Input: part model. Units: mm. Frame: model coordinates. A direction names the side the tool comes from. Coordinates: 2 decimals unless noted, no trailing zeros. Order: outer loops, then holes, each group sorted by start corner. A loop starts at its lowest first (then second) coordinate and runs counter-clockwise, first axis right, second up. Notation, with made-up numbers: (-19, 58) -> (0, 58) arc R20 cw to (0, 71) -> close; hole circle Ø6 at (55, 0.25). An arc over 180 degrees is marked (long way). Write each question's results on one line, items separated by ' | '.
```python
from build123d import *

# Parameters (mm, degrees)
ESBO_O1_W                  = 130
ESBO_O1_H                  = 40
RESSALTO_EXTRUS_O1_DEPTH   = 12
CORTE_EXTRUS_O3_DEPTH      = 70.057946682
CORTE_EXTRUS_O3_DEPTH_BACK = 4
CORTE_EXTRUS_O4_DEPTH      = 70.057946682
CORTE_EXTRUS_O4_DEPTH_BACK = 4
ESBO_O5_R                  = 4.5
CORTE_EXTRUS_O5_DEPTH      = 69.476273263
ESBO_O7_W                  = 15
ESBO_O7_H                  = 40
RESSALTO_EXTRUS_O2_DEPTH   = 50
ESBO_O8_W                  = 10
ESBO_O8_H                  = 40
RESSALTO_EXTRUS_O3_DEPTH   = 50
ESBO_O9_W                  = 40
ESBO_O9_H                  = 8
RESSALTO_EXTRUS_O4_DEPTH   = 20
ESBO_O10_R                 = 4
CORTE_EXTRUS_O6_DEPTH      = 20
CORTE_EXTRUS_O7_DEPTH      = 20
ESBO_O12_R                 = 6
CORTE_EXTRUS_O8_DEPTH      = 20


with BuildPart() as part:
    # Esboço1 → Ressalto-extrusão1 (new body)
    with BuildSketch(Plane(origin=(0, 0, 0), x_dir=(1, 0, 0), z_dir=(0, 1, 0))):
        Rectangle(ESBO_O1_W, ESBO_O1_H)
    extrude(amount=RESSALTO_EXTRUS_O1_DEPTH)

    # Esboço3 → Corte-extrusão3 (cut, two sides: drawn at the far end of the back side and taken through both)
    with BuildSketch(Plane(origin=(0, 12, 0), x_dir=(1, 0, 0), z_dir=(0, 1, 0)).offset(-CORTE_EXTRUS_O3_DEPTH_BACK)):
        with BuildLine():
            Line((-52, 13), (-65, 13))
            Line((-65, 13), (-65, -13))
            Line((-65, -13), (-52, -13))
            ThreePointArc((-52, -13), (-39, 0), (-52, 13))
        make_face()
    extrude(amount=CORTE_EXTRUS_O3_DEPTH + CORTE_EXTRUS_O3_DEPTH_BACK, mode=Mode.SUBTRACT)

    # Esboço4 → Corte-extrusão4 (cut, two sides: drawn at the far end of the back side and taken through both)
    with BuildSketch(Plane(origin=(0, 12, 0), x_dir=(1, 0, 0), z_dir=(0, 1, 0)).offset(-CORTE_EXTRUS_O4_DEPTH_BACK)):
        with BuildLine():
            Line((343.246155611, 13), (65, 13))
            Line((65, 13), (52, 13))
            ThreePointArc((52, 13), (39, 0), (52, -13))
            Line((52, -13), (65, -13))
            Line((65, -13), (343.246155611, -13))
            Line((343.246155611, -13), (899.738466833, -13))
            Line((899.738466833, -13), (899.738466833, 13))
            Line((899.738466833, 13), (343.246155611, 13))
        make_face()
    extrude(amount=CORTE_EXTRUS_O4_DEPTH + CORTE_EXTRUS_O4_DEPTH_BACK, mode=Mode.SUBTRACT)

    # Esboço5 → Corte-extrusão5 (cut, through all)
    with BuildSketch(Plane(origin=(0, 8, 0), x_dir=(1, 0, 0), z_dir=(0, 1, 0))):
        with Locations(Location((-52, 0, 0), (0, 0, 270))):
            Circle(ESBO_O5_R)
        with Locations(Location((52, 0, 0), (0, 0, 270))):
            Circle(ESBO_O5_R)
    extrude(amount=-CORTE_EXTRUS_O5_DEPTH, mode=Mode.SUBTRACT)

    # Esboço7 → Ressalto-extrusão2 (add)
    with BuildSketch(Plane(origin=(0, 12, 0), x_dir=(1, 0, 0), z_dir=(0, 1, 0))):
        with Locations((-27.5, 0)):
            Rectangle(ESBO_O7_W, ESBO_O7_H)
    extrude(amount=RESSALTO_EXTRUS_O2_DEPTH)

    # Esboço8 → Ressalto-extrusão3 (add)
    with BuildSketch(Plane(origin=(0, 12, 0), x_dir=(1, 0, 0), z_dir=(0, 1, 0))):
        with Locations((30, 0)):
            Rectangle(ESBO_O8_W, ESBO_O8_H)
    extrude(amount=RESSALTO_EXTRUS_O3_DEPTH)

    # Esboço9 → Ressalto-extrusão4 (add)
    with BuildSketch(Plane.ZY.offset(-25)):
        with Locations((0, 58)):
            Rectangle(ESBO_O9_W, ESBO_O9_H)
    extrude(amount=RESSALTO_EXTRUS_O4_DEPTH)

    # Esboço10 → Corte-extrusão6 (cut)
    with BuildSketch(Plane(origin=(0, 62, 0), x_dir=(1, 0, 0), z_dir=(0, 1, 0))):
        with Locations(Location((20, 0, 0), (0, 0, 270))):
            Circle(ESBO_O10_R)
    extrude(amount=-CORTE_EXTRUS_O6_DEPTH, mode=Mode.SUBTRACT)

    # Esboço11 → Corte-extrusão7 (cut)
    with BuildSketch(Plane.ZY.offset(35)):
        with BuildLine():
            Line((-20, 37), (-20, 62))
            Line((-20, 62), (20, 62))
            Line((20, 62), (20, 37))
            ThreePointArc((20, 37), (0, 57), (-20, 37))
        make_face()
    extrude(amount=-CORTE_EXTRUS_O7_DEPTH, mode=Mode.SUBTRACT)

    # Esboço12 → Corte-extrusão8 (cut)
    with BuildSketch(Plane.ZY.offset(35)):
        with Locations((0, 37)):
            Circle(ESBO_O12_R)
    extrude(amount=-CORTE_EXTRUS_O8_DEPTH, mode=Mode.SUBTRACT)


solid = part.part
```
(1) Cut plane B-B, the plane z = 0. Count the separate pieces of the cut face and the enclosed holes in it, plus the area to 3 significant figures.
Return value:
separate pieces: 5 | enclosed holes: 0 | area: 2,300 mm2
(2) Mould query, pull axis Z, two halves, no side actions, for faces 1 (the face through (58, 10, 13)), 2 (the face through (0, 10, -20)), 3 (the face through (59, 10, -13)), 4 (the face through (-1, 0, 0)). Classes: +Z half, -Z half, draft (parallel to the pull), parting line (faces both ways), or undercut.
Return value:
face 1: undercut | face 2: -Z half | face 3: undercut | face 4: draft
(3) Cut plane C-C, the plane x = -30. Return loops of the section in (y, z).
Return value:
outline: (0, -20) -> (37, -20) arc R20 ccw to (37, 20) -> (0, 20) -> close; hole circle Ø12 at (37, 0)
(4) Line query: line 1 along X through (y, z) = (5.5, 0); line 2 along Y through (x, z) = (5.5, -14); line 3 along X through (y, z) = (12.5, 12). Output: solid intervals per line, ascending. Write a range as from..to.
Return value:
line 1: -65..-56.5, -47.5..47.5, 56.5..65 | line 2: 0..12, 54..62 | line 3: -35..-20, 25..35
(5) Pin query (flat end, axial travel): P1, Ø16, axis at x = 13.5, z = 0, coming from the -Y side; P2, Ø1.5, axis at y = 9.5, z = -7, coming from the -X side; P3, Ø12, axis at y = 43, z = 4.5, coming from the -X side; P4, Ø5, axis at y = 15.5, z = 6.5, coming from the +X side. Return the tip coordinate at first contact, or that it passes through.
Return value:
P1: y = 0 | P2: x = -41.56 | P3: x = -35 | P4: x = 35
(6) Reachability of faces 5 (the face through (-20, 29, 0)), 6 (the face through (58, 8, 0)), 7 (the face through (35, 37, 0)), 8 (the face through (25, 33, 0)), 9 (the face through (23.966, 58.056, -0.521)) from +Z, -Z, +X, -X, +Y, -Y: full face, straight path, thin tool, end or side. Return the list, or none.
Return value:
face 5: +Z, -Z, +Y | face 6: +X, +Y | face 7: +Z, -Z, +X, +Y | face 8: +Z, -Z | face 9: +Y
(7) Cut plane D-D, the plane x = 55. Return loops of the section in (y, z), plus the area to 3 significant figures.
Return value:
outline: (0, -20) -> (12, -20) -> (12, -13) -> (8, -13) -> (8, -3.35) -> (0, -3.35) -> close; (0, 3.35) -> (8, 3.35) -> (8, 13) -> (12, 13) -> (12, 20) -> (0, 20) -> close | area: 322 mm2
(8) Cut plane A-A, the plane x = 20. Return loops of the section in (y, z).
Return value:
outline: (0, -20) -> (12, -20) -> (12, 20) -> (0, 20) -> close; (54, -20) -> (62, -20) -> (62, -4) -> (54, -4) -> close; (54, 4) -> (62, 4) -> (62, 20) -> (54, 20) -> close
